Source: three-view drawing plus pictorial views. Frame: mm from the lowest corner of the part. A direction names the side the tool comes from. Coordinates: 2 decimals unless noted, no trailing zeros. Loops run counter-clockwise (first coordinate to the right, second up) from the corner with the lowest first, then second, coordinate; pieces in that order, holes last. Notation, with made-up numbers: M 38,-2.75 L 52,-2.75 A28 cw 52,15.25 Z; hole C 67.5,60 d4. An arc over 180 degrees is marked long. Write each question's results on one line, items separated by ' | '. Start each with the question number.
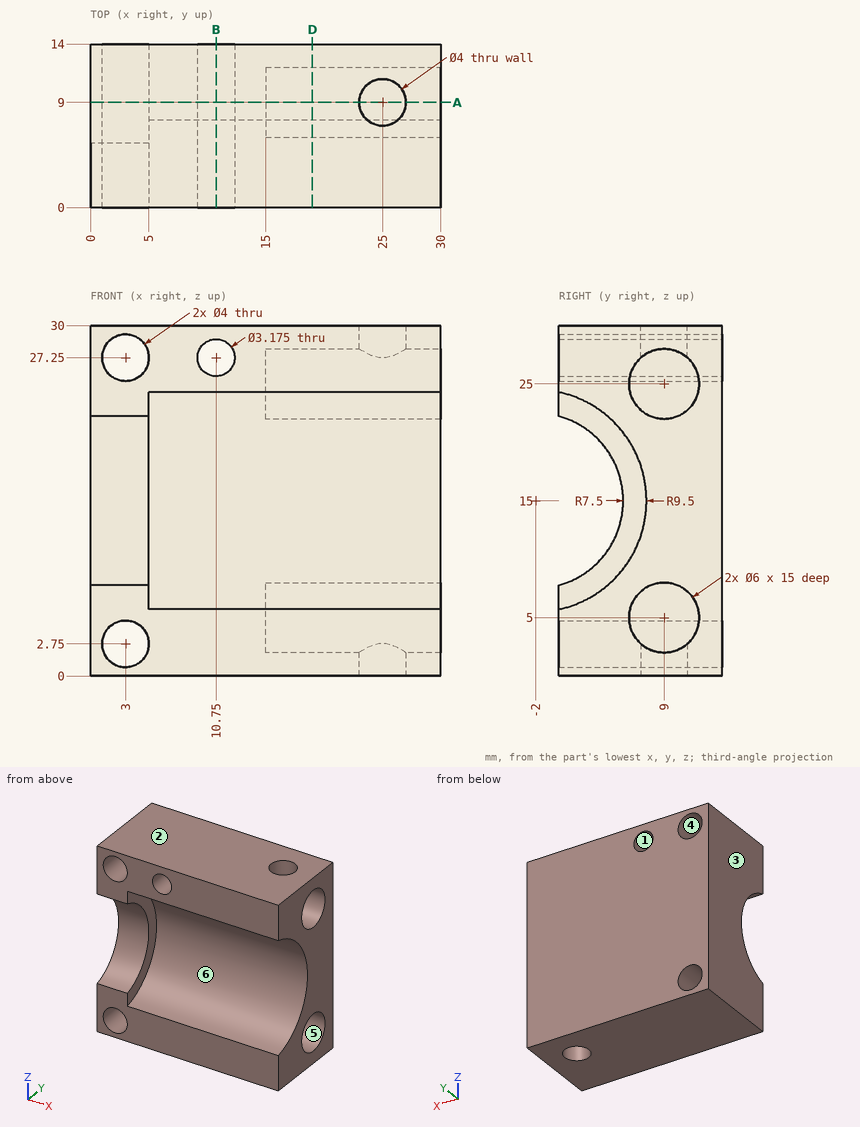
Item 1: Section D-D, the plane x = 19. Return loops of the section in (y, z), plus the area to 3 significant figures.
Item 2: Contact query for flat-ended pins moving along their axis: P1, Ø5, axis at y = 9, z = 5, coming from the +X side; P2, Ø3.5, axis at x = 25, y = 9, coming from the -Z side; P3, Ø2.5, axis at y = 4, z = 15, coming from the +X side; P4, Ø3.5, axis at x = 25, y = 9, coming from the +Z side. Output: stop coordinate, or through.
Item 3: Section A-A, the plane y = 9. Count the separate pieces of the cut face and the enclosed holes in it, plus the area to 3 significant figures.
Item 4: Ray query, L1, parallel to Z at x = 3, y = 6.75; L2, parallel to Y at x = 25.75, z = 5; L3, parallel to Z at x = 20, y = 9. Return the intervals inside material, ascending. Write a range as [from, to].
Item 5: Section B-B, the plane x = 10.75. Return loops of the section in (y, z), plus the area to 4 significant figures.
Item 6: Set-up query: the marked faces 4, 5 and 6. Return all of +Z, -Z, +X, -X, +Y, -Y with unobstructed straight access to the full face (end or side cutting, diameter ignored); none if empty.
Item 7: Pull-direction query (X, two-part tool) for the marked faces 1, 2 and 3; classes: released by +X, released by -X, zero draft, split by the parting line, or undercut.
Solutions:
1) outline: M 0,0 L 14,0 L 14,30 L 0,30 L 0,24.29 A9.5 cw 0,5.71 Z; hole C 9,5 d6; hole C 9,25 d6 | area: 259 mm²
2) P1: stops at x = 15 | P2: stops at z = 7.44 | P3: passes through | P4: stops at z = 22.56
3) separate pieces: 3 | enclosed holes: 3 | area: 671 mm²
4) L1: z = [0, 0.75], [4.75, 25.25], [29.25, 30] | L2: y = [0, 6], [12, 14] | L3: z = [0, 2], [8, 22], [28, 30]
5) outline: M 0,0 L 14,0 L 14,25.66 L 0,25.66 L 0,24.29 A9.5 cw 0,5.71 Z; M 0,28.84 L 14,28.84 L 14,30 L 0,30 Z | area: 271.5 mm²
6) face 4: +Y, -Y | face 5: +X | face 6: +X, -Y
7) face 1: undercut | face 2: zero draft | face 3: released by -X
